Check sheet for the drawn part. Datum: minimum x, y, z corner. Units: mm. A direction names the side the tool comes from. Give positions to 0.01 mm unless a question says otherwise; leave off trailing zeros. Write each loop counter-clockwise with the first axis right and the second up, starting at its lowest first coordinate (ties: lowest second). Pieces come first, ordered by that corner, then holes. Notation, with made-up numbers: (-19, 65.5) - (-10, 65.5) arc R3 ccw to (-10, 70.5) - close; hole circle Ø1 at (42.5, -19). An arc over 180 degrees is marked (long way). Use a Markdown table: item, result.
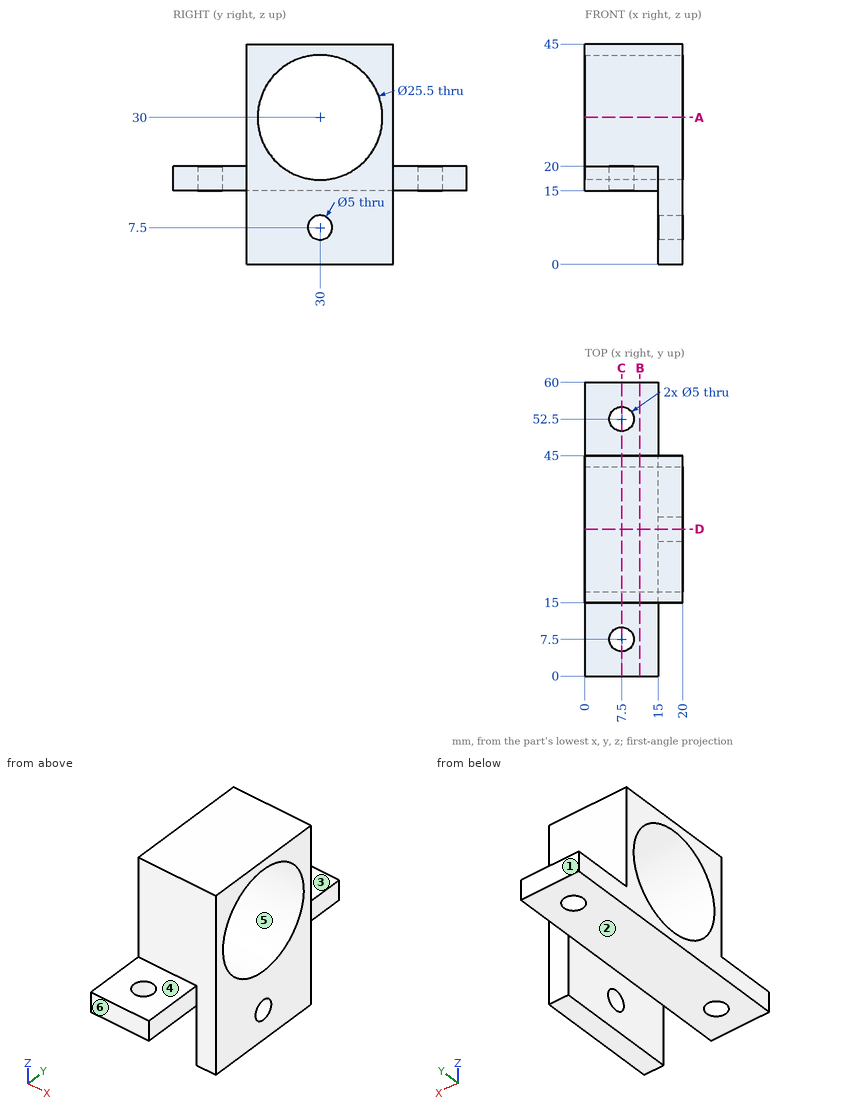
1) Set-up check for the marked faces 1, 2 and 3: record each of +Z, -Z, +X, -X, +Y, -Y from which the full face is reachable in a straight line by a thin tool's end or side.
Working result:
| item | result |
|---|---|
| face 1 | +Z, -Z, +X, -X, +Y |
| face 2 | -Z, -X, +Y, -Y |
| face 3 | +Z, +X, -X, +Y |
2) Mould release check, pull along Z, two halves, no side actions. Record for the marked faces 4, 5 and 6: pulls with the +Z half, pulls with the -Z half, needs draft (parallel to the pull), parting line crosses it, or undercut.
Working result:
| item | result |
|---|---|
| face 4 | pulls with the +Z half |
| face 5 | undercut |
| face 6 | needs draft |
3) Section check B-B on x = 11.25. Record the boundary of the cut face in (y, z).
Working result:
| item | result |
|---|---|
| outline | (0, 15) - (60, 15) - (60, 20) - (45, 20) - (45, 45) - (15, 45) - (15, 20) - (0, 20) - close; hole circle Ø25.5 at (30, 30) |
4) Section check A-A on z = 30. Record the boundary of the cut face in (x, y), then the cut area to 3 significant figures.
Working result:
| item | result |
|---|---|
| outline | (0, 15) - (20, 15) - (20, 17.25) - (0, 17.25) - close; (0, 42.75) - (20, 42.75) - (20, 45) - (0, 45) - close |
| area | 90.0 mm² |
5) Depth check by flat-ended pin: P1, Ø12, axis at x = 5, y = 51.5, coming from the +Z side; P2, Ø1.5, axis at x = 12, y = 26.5, coming from the -Z side; P3, Ø2.5, axis at y = 6, z = 17, coming from the +X side. Enter the tip coordinate at first touch or a pass-through.
Working result:
| item | result |
|---|---|
| P1 | stops at z = 20 |
| P2 | stops at z = 15 |
| P3 | stops at x = 15 |
6) Section check C-C on x = 7.5. Record the boundary of the cut face in (y, z), then the cut area to 3 significant figures.
Working result:
| item | result |
|---|---|
| outline | (0, 15) - (5, 15) - (5, 20) - (0, 20) - close; (10, 15) - (50, 15) - (50, 20) - (45, 20) - (45, 45) - (15, 45) - (15, 20) - (10, 20) - close; (55, 15) - (60, 15) - (60, 20) - (55, 20) - close; hole circle Ø25.5 at (30, 30) |
| area | 489 mm² |
7) Material ranges on L1, parallel to Y at x = 7.5, z = 16.65; L2, parallel to Y at x = 7.5, z = 18.5; L3, parallel to Y at x = 4.5, z = 30, recorded low to high. Write a range as from..to.
Working result:
| item | result |
|---|---|
| L1 | y = 0..5, 10..50, 55..60 |
| L2 | y = 0..5, 10..24.49, 35.51..50, 55..60 |
| L3 | y = 15..17.25, 42.75..45 |
8) Section check D-D on y = 30. Record the boundary of the cut face in (x, z), then the cut area to 3 significant figures.
Working result:
| item | result |
|---|---|
| outline | (0, 15) - (15, 15) - (15, 10) - (20, 10) - (20, 17.25) - (0, 17.25) - close; (0, 42.75) - (20, 42.75) - (20, 45) - (0, 45) - close; (15, 0) - (20, 0) - (20, 5) - (15, 5) - close |
| area | 140 mm² |
